Check sheet for the modelled part. Datum: model origin and axes. Units: mm. Coordinates: 2 decimals unless noted, no trailing zeros. Write each loop counter-clockwise with the first axis right and the second up, starting at its lowest first coordinate (ties: lowest second). Pieces come first, ordered by that corner, then holes. Notation, with made-up numbers: (42.5, 60.5) -> (90.5, 60.5) arc R36 ccw to (90.5, 98.5) -> close; hole circle Ø5 at (24.25, 41). An arc over 180 degrees is marked (long way). Put each result on its own line as item: value.
```python
from build123d import *

# Parameters (mm, degrees)
F1_DEPTH = 1


# Not quite as in the source:
# - ends of sketch curves that miss each other by under 0.0002 mm in the source are joined


with BuildPart() as f1:
    # F0 (on Top) → F1 (new body)
    with BuildSketch(Plane.XY):
        with BuildLine():
            ThreePointArc((31.2898730428, -1.0903693776), (36.8162528215, -2.4992396802), (41.4861883055, -5.7729976987))
            Line((41.4861883055, -5.7729976987), (42.499983, -5.772998))
            Line((42.499983, -5.772998), (42.499983, 5.772998))
            Line((42.499983, 5.772998), (-42.499983, 5.772998))
            Line((-42.499983, 5.772998), (-42.499983, -5.772998))
            Line((-42.499983, -5.772998), (-41.486188, -5.772998))
            ThreePointArc((-41.486188, -5.772998), (-36.8162528215, -2.4992396802), (-31.2898730428, -1.0903693776))
            Line((-31.2898730428, -1.0903693776), (31.2898730428, -1.0903693776))
        make_face()
        with BuildLine():
            ThreePointArc((-37.980823226, -1.9562535657), (-39.8184929613, -3.0669655752), (-41.4999834083, -4.4023685483))
            Line((-41.4999834083, -4.4023685483), (-41.499983, 3.305772))
            Line((-41.499983, 3.305772), (-37.947737, -0.508143))
            ThreePointArc((-37.947737, -0.508143), (-38.1314028467, -1.2283801993), (-37.980823226, -1.9562535657))
        make_face(mode=Mode.SUBTRACT)
        with BuildLine():
            Line((41.499983, 3.305772), (41.499983, -4.402369))
            ThreePointArc((41.499983, -4.402369), (39.8184929613, -3.0669655752), (37.980823226, -1.9562535657))
            ThreePointArc((37.980823226, -1.9562535657), (38.1314028467, -1.2283801993), (37.9477363989, -0.5081433103))
            Line((37.9477363989, -0.5081433103), (41.499983, 3.305772))
        make_face(mode=Mode.SUBTRACT)
        with BuildLine():
            Line((-31.289873, 2.077969), (-31.289873, -0.09037))
            ThreePointArc((-31.289873, -0.09037), (-33.1211344425, -0.3089644519), (-34.9175362693, -0.7263880763))
            ThreePointArc((-34.9175362693, -0.7263880763), (-35.2042200678, -0.2151094555), (-35.6513559051, 0.1639211639))
            Line((-35.6513559051, 0.1639211639), (-34.24769, 4.772998))
            Line((-34.24769, 4.772998), (-31.289873, 2.077969))
        make_face(mode=Mode.SUBTRACT)
        with BuildLine():
            Line((-37.241042, 0.200331), (-41.499983, 4.772998))
            Line((-41.499983, 4.772998), (-35.293036, 4.772998))
            Line((-35.293036, 4.772998), (-36.631091, 0.379359))
            ThreePointArc((-36.631091, 0.379359), (-36.9447562748, 0.3194512642), (-37.241042, 0.200331))
        make_face(mode=Mode.SUBTRACT)
        Polygon((-22.953359, -0.09037), (-27.06573, -0.09037), (-27.06573, 2.077969), (-25.009544, 3.951473), (-22.953359, 2.077969), align=None, mode=Mode.SUBTRACT)
        Polygon((-14.616844, -0.09037), (-18.729215, -0.09037), (-18.729215, 2.077969), (-16.67303, 3.951473), (-14.616844, 2.077969), align=None, mode=Mode.SUBTRACT)
        Polygon((-6.280329, -0.09037), (-10.392701, -0.09037), (-10.392701, 2.077969), (-8.44277, 3.854658), (-6.280329, 1.884339), align=None, mode=Mode.SUBTRACT)
        Polygon((-25.584392, 4.772998), (-28.130887, 2.456623), (-30.224716, 2.456623), (-32.771212, 4.772998), align=None, mode=Mode.SUBTRACT)
        Polygon((-19.794373, 2.456623), (-21.888201, 2.456623), (-24.434697, 4.772998), (-17.247877, 4.772998), align=None, mode=Mode.SUBTRACT)
        Polygon((-11.457858, 2.456623), (-13.551687, 2.456623), (-16.098182, 4.772998), (-8.911362, 4.772998), align=None, mode=Mode.SUBTRACT)
        Polygon((-3.121343, 2.262993), (-5.215172, 2.262993), (-7.974534, 4.772998), (-0.361981, 4.772998), align=None, mode=Mode.SUBTRACT)
        Polygon((0, -0.09037), (-2.056186, -0.09037), (-2.056186, 1.884339), (0, 3.757843), (2.056186, 1.884339), (2.056186, -0.09037), align=None, mode=Mode.SUBTRACT)
        Polygon((10.392701, 2.077969), (10.392701, -0.09037), (6.280329, -0.09037), (6.280329, 1.884339), (8.44277, 3.854658), align=None, mode=Mode.SUBTRACT)
        Polygon((18.729215, 2.077969), (18.729215, -0.09037), (14.616844, -0.09037), (14.616844, 2.077969), (16.67303, 3.951473), align=None, mode=Mode.SUBTRACT)
        Polygon((27.06573, 2.077969), (27.06573, -0.09037), (22.953359, -0.09037), (22.953359, 2.077969), (25.009544, 3.951473), align=None, mode=Mode.SUBTRACT)
        with BuildLine():
            Line((31.289873, -0.09037), (31.289873, 2.077969))
            Line((31.289873, 2.077969), (34.24769, 4.772998))
            Line((34.24769, 4.772998), (35.651356, 0.163921))
            ThreePointArc((35.651356, 0.163921), (35.2042200678, -0.2151094555), (34.9175353631, -0.7263887799))
            ThreePointArc((34.9175353631, -0.7263887799), (33.1211344425, -0.3089644519), (31.289873, -0.09037))
        make_face(mode=Mode.SUBTRACT)
        with BuildLine():
            Line((35.293036, 4.772998), (41.499983, 4.772998))
            Line((41.499983, 4.772998), (37.241042, 0.200331))
            ThreePointArc((37.241042, 0.200331), (36.9447562748, 0.3194512642), (36.6310910035, 0.3793590379))
            Line((36.6310910035, 0.3793590379), (35.293036, 4.772998))
        make_face(mode=Mode.SUBTRACT)
        Polygon((7.974534, 4.772998), (5.215172, 2.262993), (3.121343, 2.262993), (0.361981, 4.772998), align=None, mode=Mode.SUBTRACT)
        Polygon((16.098182, 4.772998), (13.551687, 2.456623), (11.457858, 2.456623), (8.911362, 4.772998), align=None, mode=Mode.SUBTRACT)
        Polygon((24.434697, 4.772998), (21.888201, 2.456623), (19.794373, 2.456623), (17.247877, 4.772998), align=None, mode=Mode.SUBTRACT)
        Polygon((32.771212, 4.772998), (30.224716, 2.456623), (28.130887, 2.456623), (25.584392, 4.772998), align=None, mode=Mode.SUBTRACT)
    extrude(amount=F1_DEPTH)


solid = f1.part
```
Q1. Material ranges on line 1 along Y through (x, z) = (-4.5, 0.85); line 2 along Y through (x, z) = (26.5, 0.85); line 3 along X through (y, z) = (-2.5, 0.45), recorded low to high.
Recorded:
line 1: y = -1.09 to 2.26, 4.77 to 5.77
line 2: y = -1.09 to -0.09, 2.59 to 3.94, 4.77 to 5.77
line 3: x = -42.5 to -41.5, -38.95 to -36.82, 36.82 to 38.95, 41.5 to 42.5
Q2. Mould release check, pull along Y, two halves, no side actions. Record for faces 1 (the flat face through (-26.052, 3.002, 0.493)), 2 (the cylindrical face through (36.743, -2.466, 0.493)), 3 (the flat face through (26.02, 3.03, 0.49)), 4 (the flat face through (-3, 2, 1)): released by +Y, released by -Y, zero draft, split by the parting line, or undercut.
Recorded:
face 1: undercut
face 2: released by -Y
face 3: undercut
face 4: zero draft
Q3. Cross-section at B-B (x = -32). Record the cut outline in (y, z) (3 decimals).
Recorded:
outline: (-1.155, 0) -> (-0.151, 0) -> (-0.151, 1) -> (-1.155, 1) -> close; (2.725, 0) -> (4.071, 0) -> (4.071, 1) -> (2.725, 1) -> close; (4.773, 0) -> (5.773, 0) -> (5.773, 1) -> (4.773, 1) -> close
Q4. Cross-section at D-D (z = 0.3). State how many separate pieces and enclosed holes the cut face has, plus the area to 3 significant figures.
Recorded:
separate pieces: 1
enclosed holes: 21
area: 357 mm2
Q5. Cross-section at C-C (y = -2.75). Record the cut outline in (x, z), plus the area to 3 significant figures.
Recorded:
outline: (-42.5, 0) -> (-41.5, 0) -> (-41.5, 1) -> (-42.5, 1) -> close; (-39.35, 0) -> (-37.34, 0) -> (-37.34, 1) -> (-39.35, 1) -> close; (37.34, 0) -> (39.35, 0) -> (39.35, 1) -> (37.34, 1) -> close; (41.5, 0) -> (42.5, 0) -> (42.5, 1) -> (41.5, 1) -> close
area: 6.02 mm2
Q6. Cross-section at A-A (x = 12.5). Record the cut outline in (y, z), plus the area to 3 significant figures.
Recorded:
outline: (-1.09, 0) -> (2.46, 0) -> (2.46, 1) -> (-1.09, 1) -> close; (4.77, 0) -> (5.77, 0) -> (5.77, 1) -> (4.77, 1) -> close
area: 4.55 mm2
